Input: part model. Units: mm. Frame: model coordinates. Face numbers are marked on the shaded views. A direction names the side the tool comes from. Give positions to 0.01 mm unless a question says otherwise; leave off trailing zeros. Loops run counter-clockwise (first coordinate to the right, second up) from the corner with the lowest first, then second, coordinate; pieces in that order, holes last. Notation, with made-up numbers: (61, 31) - (95, 31) arc R11 ccw to (95, 38) - close; hole circle Ø3 at (7, -17). An arc over 180 degrees is marked (long way). Answer as a JSON object with one key per item and string values. Group by question number.
(1) Section query D-D (x = 22.5). Return loops of the section in (y, z), plus the area to 3 significant figures.
(2) Pin query (flat end, axial travel): P1, Ø4, axis at y = -16, z = 7, coming from the +X side; P2, Ø1.6, axis at y = 1.5, z = 1, coming from the +X side; P3, Ø1.5, axis at x = 39, z = 4, coming from the -Y side; P4, Ø2.5, axis at x = 9.5, z = 7, coming from the -Y side. Return the tip coordinate at first contact, or that it passes through.
(3) Access query for the marked faces 1, 2 and 3. Directions: +Z, -Z, +X, -X, +Y, -Y. A direction counts if a zero-diameter tool reaches every point of the face in a straight line with its end or side. Return the directions, or none.
(4) Section query B-B (x = 6.5). Return loops of the section in (y, z).
(5) Section query C-C (y = 16). Return loops of the section in (x, z).
(6) Section query A-A (z = 7.25). Return loops of the section in (x, y), plus the area to 3 significant figures.
(7) Mould query, pull axis X, two halves, no side actions, for the marked faces 4, 5, 6 and 7. Classes: +X half, -X half, draft (parallel to the pull), parting line (faces both ways), or undercut.
(8) Material intervals for L1, parallel to X at y = -18, z = 5.25; L2, parallel to Y at x = 8, z = 3.5; L3, parallel to Z at x = 21.5, y = 27.5, sorted ascending.
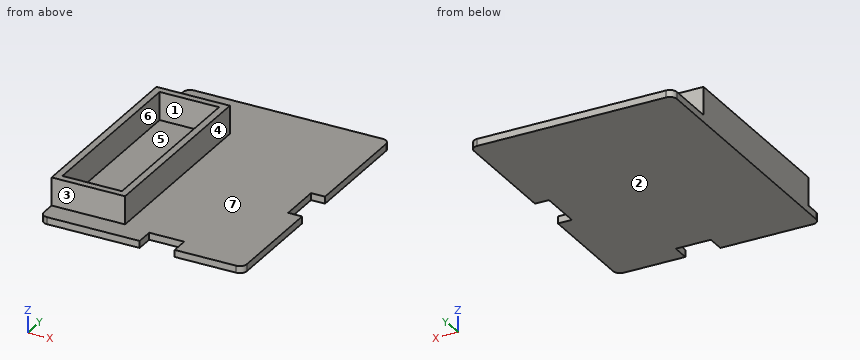
```python
from build123d import *

# Parameters (mm, degrees)
F1_DEPTH = 2
F2_DEPTH = 10
F3_T     = -2
F4_R     = 2


with BuildPart() as f1:
    # F0 (on Top) → F1 (new body)
    with BuildSketch(Plane.XY):
        Polygon((18.3934628367, 39.4180682003), (-3.6065371633, 39.4180682003), (-3.6065371633, 23.4180682003), (17.3934628367, 23.4180682003), (17.3934628367, -31.5819317997), (-3.6065371633, -31.5819317997), (-3.6065371633, -37.5819317997), (24.8428341001, -37.5819317997), (24.8428341001, -32.5819317997), (34.8428341001, -32.5819317997), (34.8428341001, -37.5819317997), (54.3934628367, -37.5819317997), (54.3934628367, -6.5819317997), (50.3934628367, -6.5819317997), (50.3934628367, 5.4180682003), (54.3934628367, 5.4180682003), (54.3934628367, 17.4180682003), (54.3934628367, 39.4180682003), (32.3934628367, 39.4180682003), align=None)
        Polygon((17.3934628367, 23.4180682003), (-3.6065371633, 23.4180682003), (-3.6065371633, 17.4180682003), (-3.6065371633, -31.5819317997), (17.3934628367, -31.5819317997), align=None)
    extrude(amount=F1_DEPTH)

    # F0 (on Top) → F2 (join)
    with BuildSketch(Plane.XY):
        Polygon((17.3934628367, 23.4180682003), (-3.6065371633, 23.4180682003), (-3.6065371633, 17.4180682003), (-3.6065371633, -31.5819317997), (17.3934628367, -31.5819317997), align=None)
    extrude(amount=F2_DEPTH)

    # F3
    f3_openings = [f1.faces().sort_by_distance(p)[0] for p in [
        (6.893463, -4.081932, 10),
    ]]
    offset(amount=F3_T, openings=f3_openings, kind=Kind.INTERSECTION)

    # F4
    f4_edges = [f1.edges().sort_by_distance(p)[0] for p in [
        (54.393463, 39.418068, 1),
        (-3.606537, 39.418068, 1),
        (54.393463, -37.581932, 1),
        (-3.606537, -37.581932, 1),
    ]]
    fillet(f4_edges, radius=F4_R)


solid = f1.part
```
Recorded:
{
 "1": {"outline": "(-37.58, 0) - (39.42, 0) - (39.42, 2) - (-37.58, 2) - close", "area": "154 mm^2"},
 "2": {"P1": "stops at x = 17.39", "P2": "stops at x = 50.39", "P3": "passes through", "P4": "stops at y = -31.58"},
 "3": {"face 1": "+Z", "face 2": "-Z, +X, -X, +Y, -Y", "face 3": "+Z, +X, -X, -Y"},
 "4": {"outline": "(-37.58, 0) - (39.42, 0) - (39.42, 2) - (23.42, 2) - (23.42, 10) - (21.42, 10) - (21.42, 2) - (-29.58, 2) - (-29.58, 10) - (-31.58, 10) - (-31.58, 2) - (-37.58, 2) - close"},
 "5": {"outline": "(-3.61, 0) - (54.39, 0) - (54.39, 2) - (17.39, 2) - (17.39, 10) - (15.39, 10) - (15.39, 2) - (-1.61, 2) - (-1.61, 10) - (-3.61, 10) - close"},
 "6": {"outline": "(-3.61, -31.58) - (17.39, -31.58) - (17.39, 23.42) - (-3.61, 23.42) - close; hole (-1.61, -29.58) - (15.39, -29.58) - (15.39, 21.42) - (-1.61, 21.42) - close", "area": "288 mm^2"},
 "7": {"face 4": "+X half", "face 5": "undercut", "face 6": "undercut", "face 7": "draft"},
 "8": {"L1": "x = -3.61 to -1.61, 15.39 to 17.39", "L2": "y = -31.58 to -29.58, 21.42 to 23.42", "L3": "z = 0 to 2"}
}
